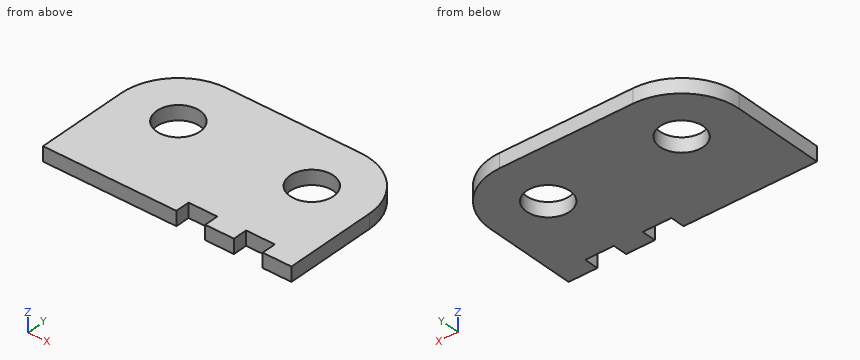
```python
from build123d import *

# Parameters (mm, degrees)
SKETCH1_R           = 4.7625
BOSS_EXTRUDE1_DEPTH = 3.175
SKETCH2_W           = 6.35
SKETCH2_H           = 3.175
CUT_EXTRUDE1_DEPTH  = 3.175


with BuildPart() as part:
    # Sketch1 → Boss-Extrude1 (new body)
    with BuildSketch(Plane.XY):
        with BuildLine():
            Line((33.387675642, 20.35683), (33.387675642, 0))
            Line((33.387675642, 0), (-21.476324358, 0))
            Line((-21.476324358, 0), (-21.476324358, 20.35683))
            ThreePointArc((-21.476324358, 20.35683), (-17.756580479, 29.337086121), (-8.776324358, 33.05683))
            Line((-8.776324358, 33.05683), (20.687675642, 33.05683))
            ThreePointArc((20.687675642, 33.05683), (29.667931764, 29.337086121), (33.387675642, 20.35683))
        make_face()
        with Locations((20.687675642, 20.35683)):
            Circle(SKETCH1_R, mode=Mode.SUBTRACT)
        with Locations((-8.776324358, 20.35683)):
            Circle(SKETCH1_R, mode=Mode.SUBTRACT)
    extrude(amount=BOSS_EXTRUDE1_DEPTH)

    # Sketch2 → Cut-Extrude1 (cut)
    with BuildSketch(Plane.XZ):
        with Locations((23.862675642, 1.5875)):
            Rectangle(SKETCH2_W, SKETCH2_H)
        with Locations((11.162675642, 1.5875)):
            Rectangle(SKETCH2_W, SKETCH2_H)
    extrude(amount=-CUT_EXTRUDE1_DEPTH, mode=Mode.SUBTRACT)


solid = part.part
```
Geometry check sheet. Reference: the model listing, model coordinates, mm. Coordinates: 2 decimals unless noted, no trailing zeros. Loops run counter-clockwise (first coordinate to the right, second up) from the corner with the lowest first, then second, coordinate; pieces in that order, holes last. Notation, with made-up numbers: (80.25, -3.75) - (91.25, -3.75) arc R30 cw to (91.25, 30.25) - close; hole circle Ø11 at (5, 86). An arc over 180 degrees is marked (long way). One line per item, written item: value. Start each with the question number.
(1) Cross-section at C-C on x = 18. Enter the section's corners in (y, z) (3 decimals), plus the area to 3 significant figures.
(2) Cross-section at A-A on y = 2.5. Enter the section's corners in (x, z) (3 decimals).
(3) Cross-section at B-B on z = 2.1. Enter the section's corners in (x, y) (1 decimal).
(4) Material ranges on line 1 (X direction, y = 16, z = 2.4); line 2 (X direction, y = 22, z = 2.2); line 3 (Y direction, x = 9, z = 0.3) (3 decimals), recorded low to high. Write a range as [from, to].
(5) Cross-section at D-D on x = -7.5. Enter the section's corners in (y, z) (3 decimals).
(6) Depth check by flat-ended pin: P1, Ø1, axis at y = 23, z = 1.5, coming from the +X side. Enter the tip coordinate at first touch or a pass-through.
Results below:
1. outline: (0, 0) - (16.425, 0) - (16.425, 3.175) - (0, 3.175) - close; (24.288, 0) - (33.057, 0) - (33.057, 3.175) - (24.288, 3.175) - close
1. area: 80.0 mm2
2. outline: (-21.476, 0) - (7.988, 0) - (7.988, 3.175) - (-21.476, 3.175) - close; (14.338, 0) - (20.688, 0) - (20.688, 3.175) - (14.338, 3.175) - close; (27.038, 0) - (33.388, 0) - (33.388, 3.175) - (27.038, 3.175) - close
3. outline: (-21.5, 0) - (8, 0) - (8, 3.2) - (14.3, 3.2) - (14.3, 0) - (20.7, 0) - (20.7, 3.2) - (27, 3.2) - (27, 0) - (33.4, 0) - (33.4, 20.4) arc R12.7 ccw to (20.7, 33.1) - (-8.8, 33.1) arc R12.7 ccw to (-21.5, 20.4) - close; hole circle Ø9.5 at (-8.8, 20.4); hole circle Ø9.5 at (20.7, 20.4)
4. line 1: x = [-21.48, -10.7], [-6.85, 18.76], [22.61, 33.39]
4. line 2: x = [-21.37, -13.25], [-4.31, 16.22], [25.16, 33.28]
4. line 3: y = [3.175, 33.057]
5. outline: (0, 0) - (15.769, 0) - (15.769, 3.175) - (0, 3.175) - close; (24.945, 0) - (33.057, 0) - (33.057, 3.175) - (24.945, 3.175) - close
6. P1: stops at x = 33.21
